Geometry check sheet. Reference: the model listing, model coordinates, mm. Face numbers are marked on the shaded views. A direction names the side the tool comes from. Give positions to 0.01 mm unless a question says otherwise; leave off trailing zeros. Loops run counter-clockwise (first coordinate to the right, second up) from the corner with the lowest first, then second, coordinate; pieces in that order, holes last. Notation, with made-up numbers: (-20.75, 78) - (0.25, 78) arc R30 ccw to (0.25, 108) - close; hole circle Ø10 at (7, -36.75). An arc over 180 degrees is marked (long way). One line per question, with ' | ' between items. Start each with the question number.
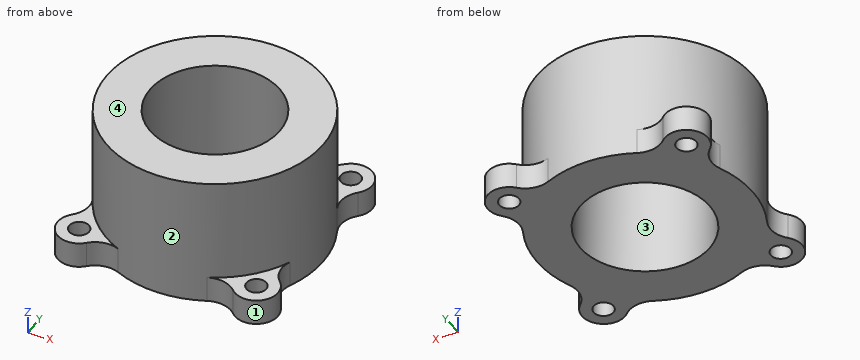
from build123d import *

# Parameters (mm, degrees)
SKETCH1_R           = 25
SKETCH1_R_2         = 15
BOSS_EXTRUDE1_DEPTH = 30
SKETCH2_R           = 5
SKETCH2_R_2         = 2.3
BOSS_EXTRUDE2_DEPTH = 6
FILLET1_R           = 6


with BuildPart() as part:
    # Sketch1 → Boss-Extrude1 (new body)
    with BuildSketch(Plane.XY):
        Circle(SKETCH1_R)
        Circle(SKETCH1_R_2, mode=Mode.SUBTRACT)
    extrude(amount=BOSS_EXTRUDE1_DEPTH)

    # Sketch2 → Boss-Extrude2 (add)
    # profile 1 of 4: a face of its own
    with BuildSketch(Plane(origin=(0, 0, 0), x_dir=(-1, 0, 0), z_dir=(0, 0, -1))):
        with Locations((20.506096654, 20.506096654)):
            Circle(SKETCH2_R)
        with Locations((20.506096654, 20.506096654)):
            Circle(SKETCH2_R_2, mode=Mode.SUBTRACT)
    # profile 2 of 4: a face of its own
    with BuildSketch(Plane(origin=(0, 0, 0), x_dir=(-1, 0, 0), z_dir=(0, 0, -1))):
        with Locations((20.506096654, -20.506096654)):
            Circle(SKETCH2_R)
        with Locations((20.506096654, -20.506096654)):
            Circle(SKETCH2_R_2, mode=Mode.SUBTRACT)
    # profile 3 of 4: a face of its own
    with BuildSketch(Plane(origin=(0, 0, 0), x_dir=(-1, 0, 0), z_dir=(0, 0, -1))):
        with Locations((-20.506096654, -20.506096654)):
            Circle(SKETCH2_R)
        with Locations((-20.506096654, -20.506096654)):
            Circle(SKETCH2_R_2, mode=Mode.SUBTRACT)
    # profile 4 of 4: a face of its own
    with BuildSketch(Plane(origin=(0, 0, 0), x_dir=(-1, 0, 0), z_dir=(0, 0, -1))):
        with Locations((-20.506096654, 20.506096654)):
            Circle(SKETCH2_R)
        with Locations((-20.506096654, 20.506096654)):
            Circle(SKETCH2_R_2, mode=Mode.SUBTRACT)
    extrude(amount=-BOSS_EXTRUDE2_DEPTH)

    # Fillet1
    fillet1_edges = [part.edges().sort_by_distance(p)[0] for p in [
        (-19.534483911, 15.601408216, 3),
        (-15.601408216, 19.534483911, 3),
        (-15.601408216, -19.534483911, 3),
        (-19.534483911, -15.601408216, 3),
        (19.534483911, -15.601408216, 3),
        (15.601408216, -19.534483911, 3),
        (15.601408216, 19.534483911, 3),
        (19.534483911, 15.601408216, 3),
    ]]
    fillet(fillet1_edges, radius=FILLET1_R)


solid = part.part
(1) Tool access check on the marked faces 1 and 2. Record the directions out of +Z, -Z, +X, -X, +Y, -Y that give a thin tool (end or side, any length) a straight path to the whole face; none if there is none.
(2) Depth check by flat-ended pin: pin 1 Ø7.5 at (x, y) = (-20.51, 20.51) entering from +Z; pin 2 Ø8 at (x, z) = (12.5, 13) entering from +Y; pin 3 Ø12 at (x, z) = (5.5, 15) entering from -Y; pin 4 Ø3.5 at (x, y) = (20.51, 20.51) entering from +Z. Enter the tip coordinate at first touch or a pass-through.
(3) Material ranges on line 1 (Y direction, x = -0.5, z = 13.5) (3 decimals); line 2 (Y direction, x = 3, z = 9.5); line 3 (X direction, y = 2, z = 23), recorded low to high.
(4) Section check A-A, the plane x = 0. Record the boundary of the cut face in (y, z).
(5) Mould release check, pull along Y, two halves, no side actions. Record for the marked faces 3 and 4: pulls with the +Y half, pulls with the -Y half, needs draft (parallel to the pull), parting line crosses it, or undercut.
(6) Section check C-C, the plane x = 20. Record the boundary of the cut face in (y, z).
(7) Section check B-B, the plane y = -9. Record the boundary of the cut face in (x, z), and give its area (3 significant figures).
(8) Section check D-D, the plane z = 15. Record the boundary of the cut face in (x, y), and give its area (3 significant figures).
Numbers:
1) face 1: +Z, -Z | face 2: +Z
2) pin 1: z = 6 | pin 2: y = 23.51 | pin 3: y = -25 | pin 4: through
3) line 1: -24.995 to -14.992, 14.992 to 24.995 | line 2: -24.82 to -14.7, 14.7 to 24.82 | line 3: -24.92 to -14.87, 14.87 to 24.92
4) outline: (-25, 0) - (-15, 0) - (-15, 30) - (-25, 30) - close; (15, 0) - (25, 0) - (25, 30) - (15, 30) - close
5) face 3: undercut | face 4: needs draft
6) outline: (-25.48, 0) - (-22.75, 0) - (-22.75, 6) - (-25.48, 6) - close; (-18.26, 0) - (18.26, 0) - (18.26, 6) - (15, 6) - (15, 30) - (-15, 30) - (-15, 6) - (-18.26, 6) - close; (22.75, 0) - (25.48, 0) - (25.48, 6) - (22.75, 6) - close
7) outline: (-23.32, 0) - (-12, 0) - (-12, 30) - (-23.32, 30) - close; (12, 0) - (23.32, 0) - (23.32, 30) - (12, 30) - close | area: 679 mm^2
8) outline: circle Ø50 at (0, 0); hole circle Ø30 at (0, 0) | area: 1,260 mm^2
